Work out the finished part from the listing and answer in its coordinate system (mm). Round coordinates to 2 decimals unless told otherwise and drop trailing zeros. Write each loop counter-clockwise with the first axis right and the second up, starting at its lowest first coordinate (ties: lowest second). Pieces come first, ordered by that corner, then holes.
1. Straight lines are drawn through the part: probe 1 along Y at (x, z) = (9.5, -0.6); probe 2 along Y at (x, z) = (-24.5, -0.2); probe 3 along X at (y, z) = (12.5, 0.1). For each, find the intervals that lie inside material, in ascending order.
2. Find section A-A (z = -0.3). Write down the section's boundary in (x, y), and give its area (3 significant figures).
3. Find section B-B (y = 16). Write down the section's boundary in (x, z) (3 decimals).
4. Find section C-C (x = 20.5). Write down the section's boundary in (y, z) (3 decimals).
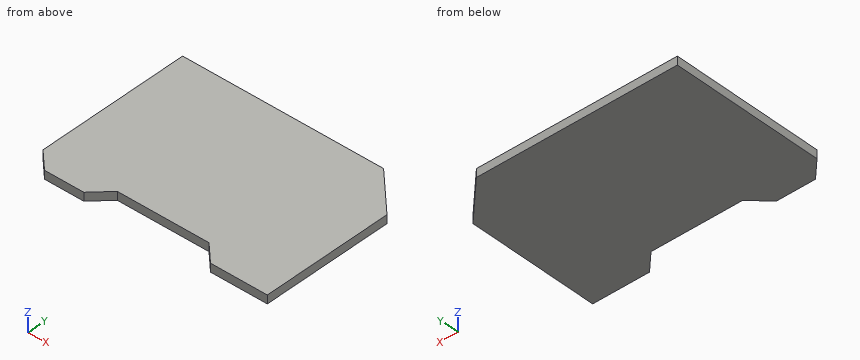
Autodesk Inventor part; units mm, degrees
ref_plane "YZ Plane" through (0, 0, 0) normal (1, 0, 0) x (0, 1, 0)
ref_plane "XZ Plane" through (0, 0, 0) normal (0, 1, 0) x (-1, 0, 0)
ref_plane "XY Plane" through (0, 0, 0) normal (0, 0, 1) x (1, 0, 0)
sketch "Sketch1" plane through (0, 0, 0) normal (0, 0, 1) x (1, 0, 0)
  line L0 (-23.5, -19.5) -> (27.5, -19.5)
  line L1 (27.5, -19.5) -> (27.5, 10.5)
  line L2 (18.5, 19.5) -> (-27.5, 19.5)
  line L3 (-27.5, 19.5) -> (-27.5, -15.5)
  line L4 (-27.5, -19.5) -> (27.5, 19.5) construction
  line L5 (27.5, -19.5) -> (-27.5, 19.5) construction
  line L6 (18.5, 19.5) -> (27.5, 10.5)
  line L7 (-27.5, -15.5) -> (-23.5, -19.5)
  line L8 (-14.5, -19.5) -> (-10.5, -15.5)
  line L9 (-10.5, -15.5) -> (10.5, -15.5)
  line L10 (10.5, -15.5) -> (14.5, -19.5)
  point P0 (0, 0)
  dimension "d0" = 55
  dimension "d1" = 39
  dimension "d2" = 9
  dimension "d3" = 9
  dimension "d4" = 4
  dimension "d5" = 4
  dimension "d11" = 17
  dimension "d12" = 17
extrude "Extrusion1" add sketch "Sketch1" along normal mid plane 1.91 contours L7 L3 L2 L6 L1 L0 L10 L9 L8
equation "\"d3\" = d2"
equation "\"d4\" = d5"
equation "\"d12\" = d11"
properties part number "Game_TurmoilPolicy"
Worked answers:
1. probe 1: y = -15.5 to 19.5
1. probe 2: y = -18.5 to 19.5
1. probe 3: x = -27.5 to 25.5
2. outline: (-27.5, -15.5) - (-23.5, -19.5) - (-14.5, -19.5) - (-10.5, -15.5) - (10.5, -15.5) - (14.5, -19.5) - (27.5, -19.5) - (27.5, 10.5) - (18.5, 19.5) - (-27.5, 19.5) - close
2. area: 2,000 mm2
3. outline: (-27.5, -0.955) - (22, -0.955) - (22, 0.955) - (-27.5, 0.955) - close
4. outline: (-19.5, -0.955) - (17.5, -0.955) - (17.5, 0.955) - (-19.5, 0.955) - close
